Can you work these out from the drawing? Everything is in mm from the part's minimum corner. Give positions to 0.01 mm unless a question says otherwise; leave off trailing zeros. Write each loop counter-clockwise with the first axis right and the second up, starting at its lowest first coordinate (ties: lowest second). Pieces come first, ordered by that corner, then holes. Notation, with made-up numbers: (10, 43) -> (41, 43) arc R16 cw to (41, 59) -> close; hole circle Ø3 at (22.25, 14). An arc over 180 degrees is marked (long way). Use one line per item in the form item = value.
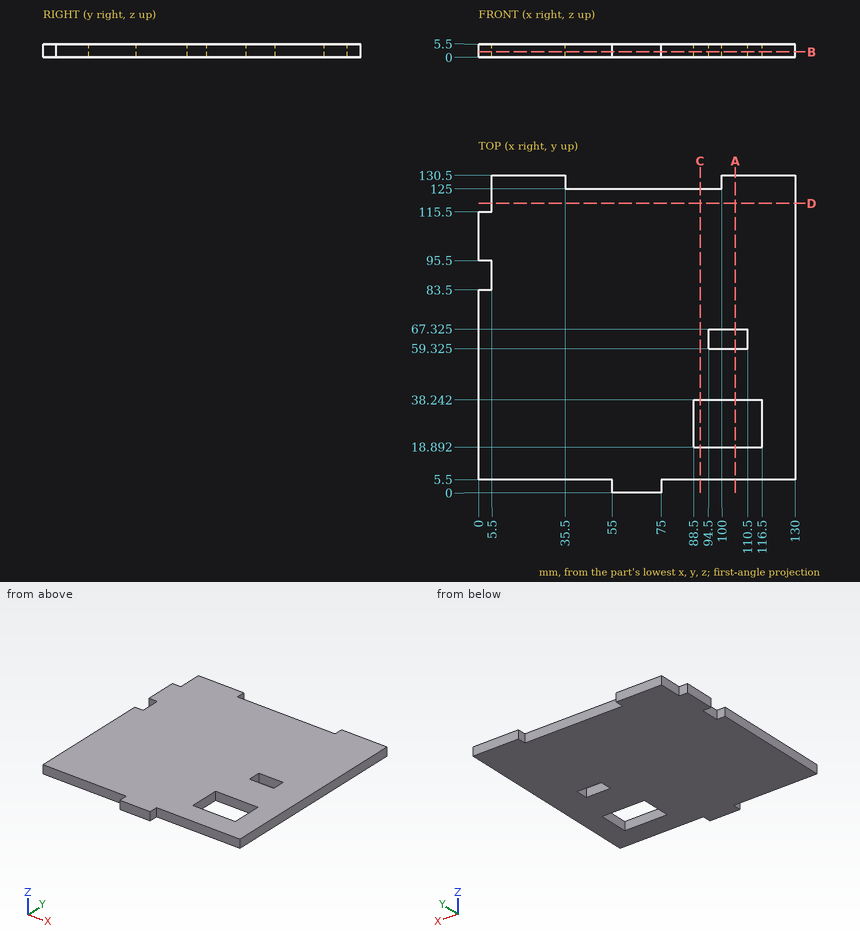
Q1. I want a section at C-C, the plane x = 91. Write out the boundary of the cut face in (y, z).
Result set:
outline = (5.5, 0) -> (18.89, 0) -> (18.89, 5.5) -> (5.5, 5.5) -> close; (38.24, 0) -> (125, 0) -> (125, 5.5) -> (38.24, 5.5) -> close
Q2. I want a section at A-A, the plane x = 105.5. Write out the boundary of the cut face in (y, z) (1 decimal), and give its area (3 significant figures).
Result set:
outline = (5.5, 0) -> (18.9, 0) -> (18.9, 5.5) -> (5.5, 5.5) -> close; (38.2, 0) -> (59.3, 0) -> (59.3, 5.5) -> (38.2, 5.5) -> close; (67.3, 0) -> (130.5, 0) -> (130.5, 5.5) -> (67.3, 5.5) -> close
area = 537 mm2
Q3. If I drill on line 1 along X through (y, z) = (116.5, 3.7); line 2 along Y through (x, z) = (93, 2.15); line 3 along Y through (x, z) = (112.5, 1.9), over which ranges is the centre line in solid material (lowest first)? Write a range as from..to.
Result set:
line_1 = 5.5..130
line_2 = 5.5..18.89, 38.24..125
line_3 = 5.5..18.89, 38.24..130.5
Q4. I want a section at B-B, the plane z = 2.25. Write out the boundary of the cut face in (x, y) (1 decimal).
Result set:
outline = (0, 5.5) -> (55, 5.5) -> (55, 0) -> (75, 0) -> (75, 5.5) -> (130, 5.5) -> (130, 130.5) -> (100, 130.5) -> (100, 125) -> (35.5, 125) -> (35.5, 130.5) -> (5.5, 130.5) -> (5.5, 115.5) -> (0, 115.5) -> (0, 95.5) -> (5.5, 95.5) -> (5.5, 83.5) -> (0, 83.5) -> close; hole (88.5, 18.9) -> (116.5, 18.9) -> (116.5, 38.2) -> (88.5, 38.2) -> close; hole (94.5, 59.3) -> (110.5, 59.3) -> (110.5, 67.3) -> (94.5, 67.3) -> close
Q5. I want a section at D-D, the plane y = 119. Write out the boundary of the cut face in (x, z), and give its area (3 significant figures).
Result set:
outline = (5.5, 0) -> (130, 0) -> (130, 5.5) -> (5.5, 5.5) -> close
area = 685 mm2
Q6. Will these pins go through, and if not, where does the flat tip stop? pin 1 Ø1.6 at (x, z) = (98.5, 2.5) entering from -Y; pin 2 Ø3 at (y, z) = (129, 2.5) entering from -X; pin 3 Ø1.6 at (y, z) = (2.5, 3) entering from +X.
Result set:
pin_1 = 5.5
pin_2 = 5.5
pin_3 = 75
